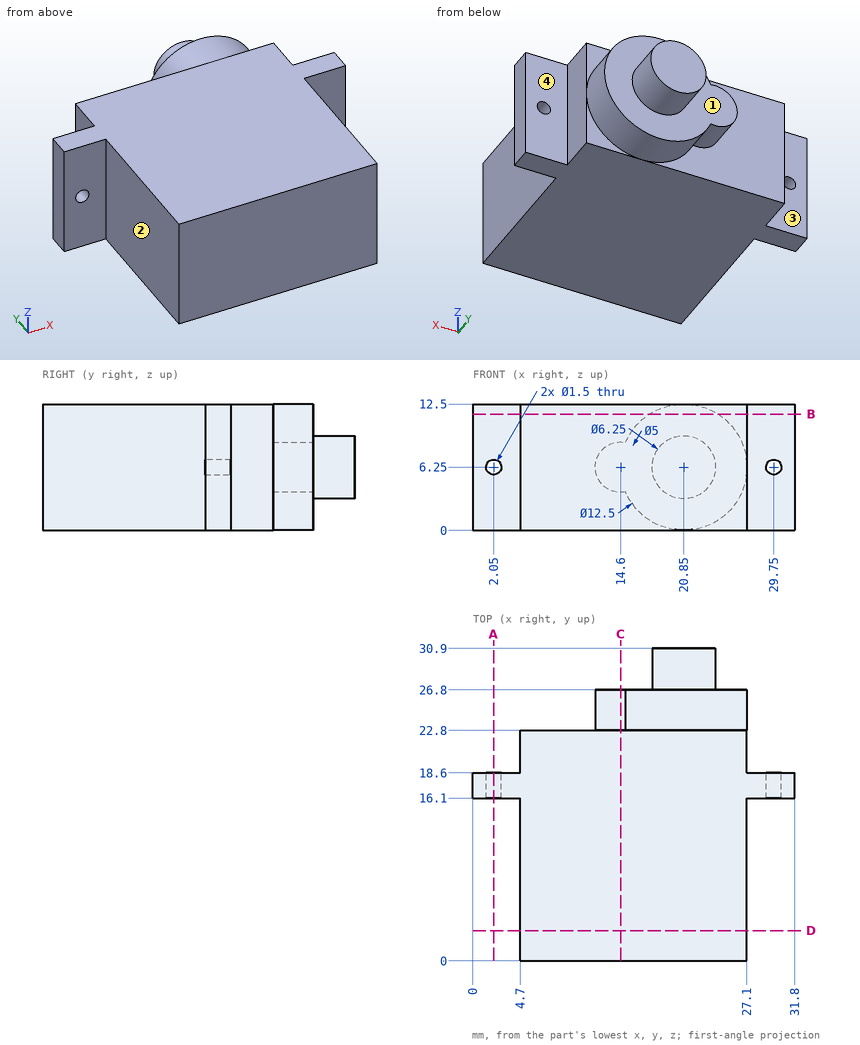
Geometry check sheet. Reference: drawing and pictorial views, mm from the part's lowest x, y, z. A direction names the side the tool comes from. Round coordinates to 2 decimals unless told otherwise and drop trailing zeros. Write each loop counter-clockwise with the first axis right and the second up, starting at its lowest first coordinate (ties: lowest second). Pieces come first, ordered by that corner, then holes. Notation, with made-up numbers: (-26.5, -10.75) -> (-6.5, -10.75) arc R11 ccw to (-6.5, -5.75) -> close; hole circle Ø9 at (-22.5, -8). An arc over 180 degrees is marked (long way). Put each result on its own line as item: value.
1) Cross-section at C-C, the plane x = 14.6. Enter the section's corners in (y, z).
Recorded:
outline: (0, 0) -> (22.8, 0) -> (22.8, 3.75) -> (26.8, 3.75) -> (26.8, 8.75) -> (22.8, 8.75) -> (22.8, 12.5) -> (0, 12.5) -> close
2) Depth check by flat-ended pin: P1, Ø1.5, axis at x = 11.5, z = 4.5, coming from the +Y side; P2, Ø2.5, axis at x = 30, z = 4.5, coming from the -Y side; P3, Ø1.4, axis at x = 2.5, z = 7.5, coming from the +Y side. Enter the tip coordinate at first touch or a pass-through.
Recorded:
P1: stops at y = 22.8
P2: stops at y = 16.1
P3: stops at y = 18.6
3) Thickness scan on probe 1 along X at (y, z) = (18.05, 6.25); probe 2 along X at (y, z) = (14, 4.5); probe 3 along Y at (x, z) = (13.5, 8). Record the ranges inside material, lowest first. Write a range as from..to.
Recorded:
probe 1: x = 0..1.3, 2.8..29, 30.5..31.8
probe 2: x = 4.7..27.1
probe 3: y = 0..26.8
4) Cross-section at B-B, the plane z = 11.5. Enter the section's corners in (x, y).
Recorded:
outline: (0, 16.1) -> (4.7, 16.1) -> (4.7, 0) -> (27.1, 0) -> (27.1, 16.1) -> (31.8, 16.1) -> (31.8, 18.6) -> (27.1, 18.6) -> (27.1, 22.8) -> (24.24, 22.8) -> (24.24, 26.8) -> (17.46, 26.8) -> (17.46, 22.8) -> (4.7, 22.8) -> (4.7, 18.6) -> (0, 18.6) -> close
5) Cross-section at D-D, the plane y = 3. Enter the section's corners in (x, z), plus the area to 3 significant figures.
Recorded:
outline: (4.7, 0) -> (27.1, 0) -> (27.1, 12.5) -> (4.7, 12.5) -> close
area: 280 mm2
6) Access from +Z, -Z, +X, -X, +Y, -Y to the whole of each face (thin tool, end or side, straight path). Record for the marked faces 1, 2, 3 and 4.
Recorded:
face 1: +Y
face 2: +Z, -Z, -X, -Y
face 3: +Z, -Z, -X, +Y
face 4: +Z, -Z, +X, +Y
7) Cross-section at A-A, the plane x = 2.05. Enter the section's corners in (y, z), plus the area to 3 significant figures.
Recorded:
outline: (16.1, 0) -> (18.6, 0) -> (18.6, 5.5) -> (16.1, 5.5) -> close; (16.1, 7) -> (18.6, 7) -> (18.6, 12.5) -> (16.1, 12.5) -> close
area: 27.5 mm2
